Here's the drawing with two shaded views (mm, measured from the low corner). I have some questions. A direction names the side the tool comes from. Round coordinates to 2 decimals unless told otherwise and drop trailing zeros. Loops run counter-clockwise (first coordinate to the right, second up) from the corner with the lowest first, then second, coordinate; pieces in that order, holes last. Notation, with made-up numbers: (66, 46) - (102, 46) arc R18 ccw to (102, 60) - close; hole circle Ø11 at (26.25, 81.25). An arc over 180 degrees is marked (long way). Use one line per item in the form item = value.
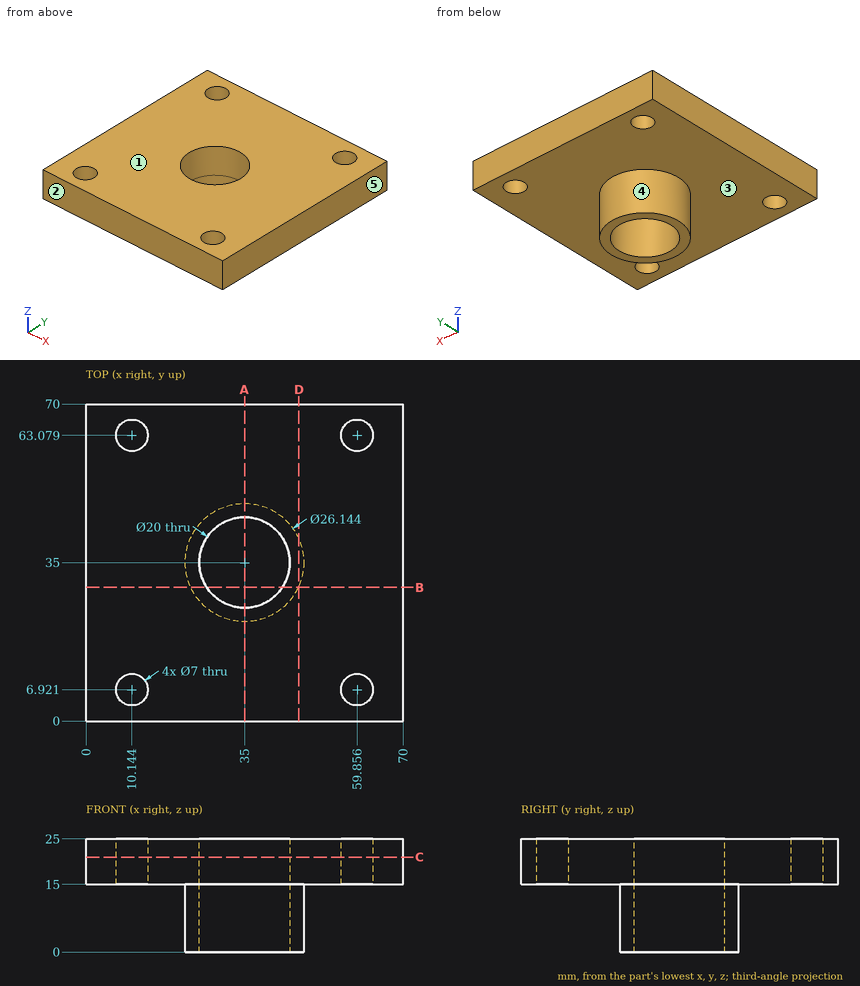
1. We'd pull the mould along Z, two halves only. Please class the marked faces 1, 2 and 3: +Z half, -Z half, draft (parallel to the pull), parting line (faces both ways), or undercut.
Solution:
face_1 = +Z half
face_2 = draft
face_3 = -Z half
2. If we section it at D-D, the plane x = 47: Write out the boundary of the cut face in (y, z) (1 decimal).
Solution:
outline = (0, 15) - (29.8, 15) - (29.8, 0) - (40.2, 0) - (40.2, 15) - (70, 15) - (70, 25) - (0, 25) - close
3. If we section it at B-B, the plane y = 29.5: Write out the boundary of the cut face in (x, z), plus the area to 3 significant figures.
Solution:
outline = (0, 15) - (23.14, 15) - (23.14, 0) - (26.65, 0) - (26.65, 25) - (0, 25) - close; (43.35, 0) - (46.86, 0) - (46.86, 15) - (70, 15) - (70, 25) - (43.35, 25) - close
area = 638 mm^2
4. For P1, Ø4, axis at x = 10.14, y = 6.92, coming from the -Z side; P2, Ø9, axis at x = 10.14, y = 63.08, coming from the +Z side; P3, Ø6, axis at x = 41, y = 10, coming from the -Z side, each with a flat end and sliding along its axis, tell me the tip position at first contact or that it passes through.
Solution:
P1 = through
P2 = 25
P3 = 15
5. Please list where these lines run through material, in increasing order: line 1 along X through (y, z) = (63, 20) (1 decimal); line 2 along Y through (x, z) = (35, 7); line 3 along Y through (x, z) = (35, 24).
Solution:
line_1 = 0 to 6.6, 13.6 to 56.4, 63.4 to 70
line_2 = 21.93 to 25, 45 to 48.07
line_3 = 0 to 25, 45 to 70
6. On a 3-axis mill with a long thin cutter (end or side, diameter ignored), from which of +Z, -Z, +X, -X, +Y, -Y can I reach the whole of each face in a straight line? I mean the marked faces 4 and 5. Say none if no direction works.
Solution:
face_4 = -Z
face_5 = +Z, -Z, +X, +Y, -Y
7. If we section it at C-C, the plane z = 21: Write out the boundary of the cut face in (x, y) (1 decimal).
Solution:
outline = (0, 0) - (70, 0) - (70, 70) - (0, 70) - close; hole circle Ø7 at (10.1, 6.9); hole circle Ø7 at (10.1, 63.1); hole circle Ø20 at (35, 35); hole circle Ø7 at (59.9, 6.9); hole circle Ø7 at (59.9, 63.1)
8. If we section it at A-A, the plane x = 35: Write out the boundary of the cut face in (y, z).
Solution:
outline = (0, 15) - (21.93, 15) - (21.93, 0) - (25, 0) - (25, 25) - (0, 25) - close; (45, 0) - (48.07, 0) - (48.07, 15) - (70, 15) - (70, 25) - (45, 25) - close
